Geometry check sheet. Reference: drawing and pictorial views, mm from the part's lowest x, y, z. A direction names the side the tool comes from. Round coordinates to 2 decimals unless told otherwise and drop trailing zeros. Write each loop counter-clockwise with the first axis right and the second up, starting at its lowest first coordinate (ties: lowest second). Pieces come first, ordered by that corner, then holes. Notation, with made-up numbers: M 44,54.25 L 60,54.25 A31 cw 60,85.25 Z; hole C 53,27.5 d6. An arc over 180 degrees is marked long. Put each result on its own line as item: value. Start each with the question number.
(1) Gauge pin test, flat ends, axial feed: pin 1 (6.5 mm diameter, centred on x = 18, y = 6, fed in from +Z); pin 2 (4 mm diameter, centred on x = 16, y = 8, fed in from -Z); pin 3 (1.5 mm diameter, centred on y = 3.5, z = 31.5, fed in from +X). Record the tip position at first contact, or that the pin passes through.
(2) Mould release check, pull along Z, two halves, no side actions. Record for the marked faces 1, 2, 3 and 4: pulls with the +Z half, pulls with the -Z half, needs draft (parallel to the pull), parting line crosses it, or undercut.
(3) Section check B-B on z = 20. Record the cut outline in (x, y), then the cut area to 3 significant figures.
(4) Section check D-D on x = 8.75. Record the cut outline in (y, z), then the cut area to 3 significant figures.
(5) Section check C-C on x = 17.75. Record the cut outline in (y, z).
(6) Tool access check on the marked faces 5 and 6. Record the directions out of +Z, -Z, +X, -X, +Y, -Y that give a thin tool (end or side, any length) a straight path to the whole face; none if there is none.
(7) Section check A-A on y = 5.5. Record the cut outline in (x, z).
(8) Material ranges on probe 1 along Z at (x, y) = (17.75, 8.75); probe 2 along Z at (x, y) = (27, 9.5); probe 3 along X at (y, z) = (1, 21.5), recorded low to high.
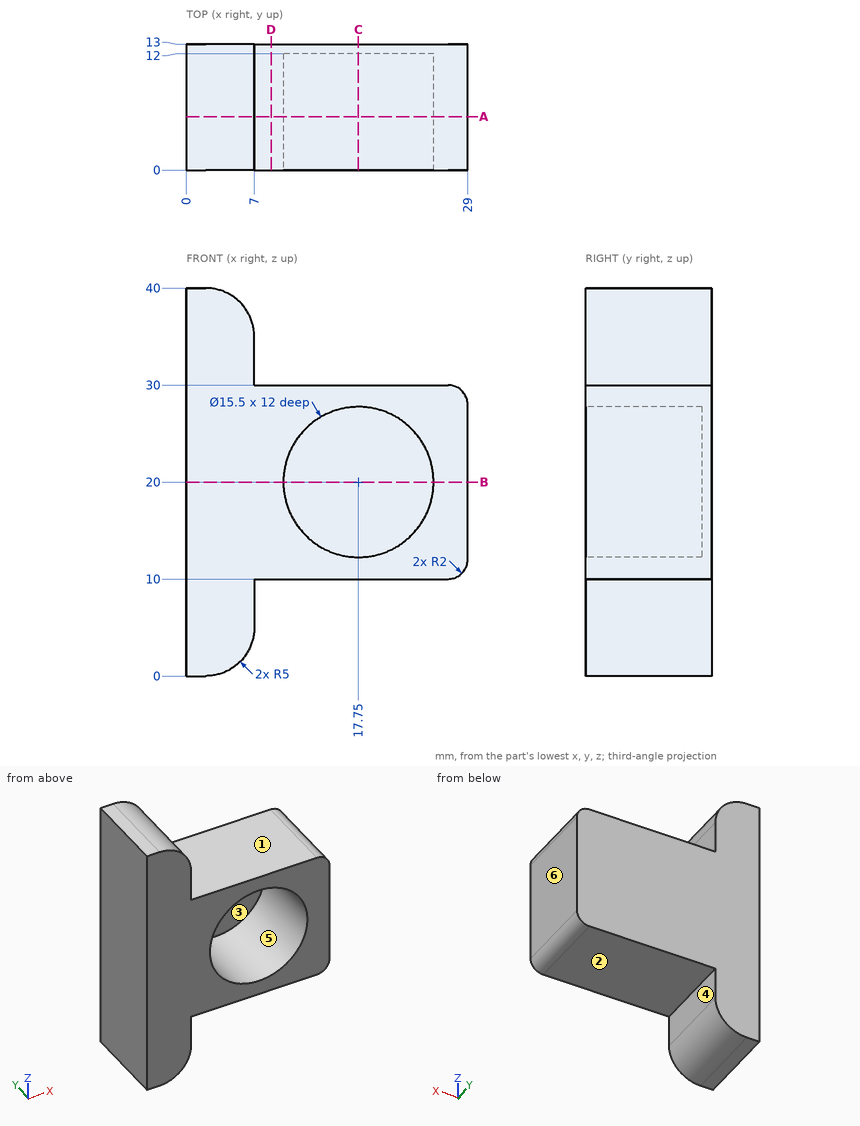
Answers follow:
1. pin 1: stops at z = 30
1. pin 2: stops at z = 10
1. pin 3: stops at x = 7
2. face 1: pulls with the +Z half
2. face 2: pulls with the -Z half
2. face 3: undercut
2. face 4: needs draft
3. outline: M 0,0 L 10,0 L 10,12 L 25.5,12 L 25.5,0 L 29,0 L 29,13 L 0,13 Z
3. area: 191 mm^2
4. outline: M 0,10 L 13,10 L 13,30 L 0,30 Z
4. area: 260 mm^2
5. outline: M 0,10 L 13,10 L 13,30 L 0,30 L 0,27.75 L 12,27.75 L 12,12.25 L 0,12.25 Z
6. face 5: -Y
6. face 6: +Z, -Z, +X, +Y, -Y
7. outline: M 0,0 L 2,0 A5 ccw 7,5 L 7,10 L 27,10 A2 ccw 29,12 L 29,28 A2 ccw 27,30 L 7,30 L 7,35 A5 ccw 2,40 L 0,40 Z; hole C 17.75,20 d15.5
8. probe 1: z = 10 to 12.25, 27.75 to 30
8. probe 2: z = 10 to 30
8. probe 3: x = 0 to 10.15, 25.35 to 29
